Model file for the job. Use its own axes, mm. A direction names the side the tool comes from. Round coordinates to 2 decimals unless told otherwise and drop trailing zeros. Loops run counter-clockwise (first coordinate to the right, second up) from the corner with the lowest first, then second, coordinate; pieces in that order, holes last. Notation, with made-up numbers: (52, 4.5) -> (65, 4.5) arc R28 ccw to (65, 39.5) -> close; hole circle Ø2 at (-34.75, -13). An arc over 180 degrees is marked (long way). Use a Markdown table: item, result.
from build123d import *

# Parameters (mm, degrees)
BOSS_EXTRUDE1_DEPTH                                 = 200
CUT_EXTRUDE1_START                                  = -200
SKETCH2_R                                           = 1.5
CUT_EXTRUDE1_DEPTH                                  = 200
CHAMFER1_SIZE                                       = 0.5
CHAMFER2_SIZE                                       = 0.5
CBORE_FOR_M4_HEX_SOCKET_HEAD_CAP_SCREW1_D           = 4.5
CBORE_FOR_M4_HEX_SOCKET_HEAD_CAP_SCREW1_CBORE_D     = 7.5
CBORE_FOR_M4_HEX_SOCKET_HEAD_CAP_SCREW1_CBORE_DEPTH = 5.3
LPATTERN1_COUNT                                     = 4
LPATTERN1_PITCH                                     = 60


with BuildPart() as part:
    # Sketch1 → Boss-Extrude1 (new body)
    with BuildSketch(Plane.XY):
        Polygon((7.5, 0), (-7.5, 0), (-7.5, 11.3), (-5.5, 11.3), (-5.5, 12.3), (-7.5, 12.3), (-7.5, 15), (7.5, 15), (7.5, 12.3), (5.5, 12.3), (5.5, 11.3), (7.5, 11.3), align=None)
    extrude(amount=BOSS_EXTRUDE1_DEPTH)

    # Sketch2 → Cut-Extrude1 (cut)
    with BuildSketch(Plane.XY.offset(200).offset(CUT_EXTRUDE1_START)):
        with Locations((-7.5, 11.8)):
            Circle(SKETCH2_R)
        with Locations((7.5, 11.8)):
            Circle(SKETCH2_R)
    extrude(amount=CUT_EXTRUDE1_DEPTH, mode=Mode.SUBTRACT)

    # Chamfer1
    chamfer1_edges = [part.edges().sort_by_distance(p)[0] for p in [
        (-7.5, 15, 100),
        (7.5, 15, 100),
    ]]
    chamfer(chamfer1_edges, length=CHAMFER1_SIZE)

    # Chamfer2
    chamfer2_edges = [part.edges().sort_by_distance(p)[0] for p in [
        (7.5, 0, 100),
        (-7.5, 0, 100),
    ]]
    chamfer(chamfer2_edges, length=CHAMFER2_SIZE)

    # CBORE for M4 Hex Socket Head Cap Screw1 (through all)
    with Locations(Plane(origin=(0, 15, 190), x_dir=(0, 0, 1), z_dir=(0, 1, 0))):
        with Locations((0, 0)):
            cbore_for_m4_hex_socket_head_cap_screw1 = CounterBoreHole(CBORE_FOR_M4_HEX_SOCKET_HEAD_CAP_SCREW1_D / 2, CBORE_FOR_M4_HEX_SOCKET_HEAD_CAP_SCREW1_CBORE_D / 2, CBORE_FOR_M4_HEX_SOCKET_HEAD_CAP_SCREW1_CBORE_DEPTH)

    # LPattern1: CBORE for M4 Hex Socket Head Cap Screw1 ×4
    with Locations(*[(0, 0, -i * LPATTERN1_PITCH) for i in range(1, LPATTERN1_COUNT)]):
        add(cbore_for_m4_hex_socket_head_cap_screw1, mode=Mode.SUBTRACT)


solid = part.part
Q1. Band-saw the part on D-D, the plane z = 52. Give the cut face in (x, y), plus the area to 3 significant figures.
Results list:
| item | result |
|---|---|
| outline | (-7.5, 0.5) -> (-7, 0) -> (7, 0) -> (7.5, 0.5) -> (7.5, 10.3) arc R1.5 cw to (6.09, 11.3) -> (5.5, 11.3) -> (5.5, 12.3) -> (6.09, 12.3) arc R1.5 cw to (7.5, 13.3) -> (7.5, 14.5) -> (7, 15) -> (-7, 15) -> (-7.5, 14.5) -> (-7.5, 13.3) arc R1.5 cw to (-6.09, 12.3) -> (-5.5, 12.3) -> (-5.5, 11.3) -> (-6.09, 11.3) arc R1.5 cw to (-7.5, 10.3) -> close |
| area | 216 mm² |
Q2. Band-saw the part on A-A, the plane z = 10. Give the cut face in (x, y), plus the area to 3 significant figures.
Results list:
| item | result |
|---|---|
| outline | (-7.5, 0.5) -> (-7, 0) -> (-2.25, 0) -> (-2.25, 9.7) -> (-3.75, 9.7) -> (-3.75, 15) -> (-7, 15) -> (-7.5, 14.5) -> (-7.5, 13.3) arc R1.5 cw to (-6.09, 12.3) -> (-5.5, 12.3) -> (-5.5, 11.3) -> (-6.09, 11.3) arc R1.5 cw to (-7.5, 10.3) -> close; (2.25, 0) -> (7, 0) -> (7.5, 0.5) -> (7.5, 10.3) arc R1.5 cw to (6.09, 11.3) -> (5.5, 11.3) -> (5.5, 12.3) -> (6.09, 12.3) arc R1.5 cw to (7.5, 13.3) -> (7.5, 14.5) -> (7, 15) -> (3.75, 15) -> (3.75, 9.7) -> (2.25, 9.7) -> close |
| area | 133 mm² |
Q3. Drill centre lines: L1, parallel to Z at x = -2, y = 8.25; L2, parallel to Z at x = 0.5, y = 8.5; L3, parallel to X at y = 11.35, z = 10. Where is each one in solid material? Low to high. Write a range as from..to.
Results list:
| item | result |
|---|---|
| L1 | z = 0..8.97, 11.03..68.97, 71.03..128.97, 131.03..188.97, 191.03..200 |
| L2 | z = 0..7.81, 12.19..67.81, 72.19..127.81, 132.19..187.81, 192.19..200 |
| L3 | x = -5.5..-3.75, 3.75..5.5 |
Q4. Band-saw the part on C-C, the plane x = 0. Give the number of separate pieces and of enclosed holes in the cut face, plus the area to 3 significant figures.
Results list:
| item | result |
|---|---|
| separate pieces | 5 |
| enclosed holes | 0 |
| area | 2,670 mm² |
Q5. Flat gauge pins, fed straight in: pin 1 (4 mm diameter, centred on x = 0, z = 190, fed in from -Y); pin 2 (1 mm diameter, centred on y = 11, z = 77, fed in from +X); pin 3 (6 mm diameter, centred on x = 0, z = 10, fed in from +Y); pin 4 (0.8 mm diameter, centred on y = 12, z = 56, fed in from -X). Where does each tip first touch, or does it go through?
Results list:
| item | result |
|---|---|
| pin 1 | passes through |
| pin 2 | stops at x = 6.75 |
| pin 3 | stops at y = 9.7 |
| pin 4 | stops at x = -6.13 |
Q6. Tool access for faces 1 (the face through (-2, 9.7, 192)), 2 (the face through (7.5, 5, 99)): list every direction of +Z, -Z, +X, -X, +Y, -Y with a clear straight run to the whole face (end or side of a thin tool).
Results list:
| item | result |
|---|---|
| face 1 | +Y |
| face 2 | +Z, -Z, +X, +Y, -Y |
Q7. Pull direction Z, two halves, no side cores. Call faces 3 (the face through (0, 8, 0)), 4 (the face through (0, 8, 200)), 5 (the face through (-2, 9.7, 132)): released by +Z, released by -Z, zero draft, split by the parting line, or undercut.
Results list:
| item | result |
|---|---|
| face 3 | released by -Z |
| face 4 | released by +Z |
| face 5 | undercut |
Q8. Band-saw the part on B-B, the plane y = 4.75. Give the cut face in (x, z), plus the area to 3 significant figures.
Results list:
| item | result |
|---|---|
| outline | (-7.5, 0) -> (7.5, 0) -> (7.5, 200) -> (-7.5, 200) -> close; hole circle Ø4.5 at (0, 10); hole circle Ø4.5 at (0, 70); hole circle Ø4.5 at (0, 130); hole circle Ø4.5 at (0, 190) |
| area | 2,940 mm² |
